Autodesk Inventor part; units mm, degrees
ref_plane "YZ Plane" through (0, 0, 0) normal (1, 0, 0) x (0, 1, 0)
ref_plane "XZ Plane" through (0, 0, 0) normal (0, 1, 0) x (-1, 0, 0)
ref_plane "XY Plane" through (0, 0, 0) normal (0, 0, 1) x (1, 0, 0)
sketch "Sketch1" plane through (0, 0, 0) normal (0, 1, 0) x (-1, 0, 0)
  line L0 (7.98, 15.9) -> (-7.98, 15.9)
  line L1 (-7.98, 15.9) -> (-7.98, -15.9)
  line L2 (-7.98, -15.9) -> (7.98, -15.9)
  line L3 (7.98, -15.9) -> (7.98, 15.9)
  line L4 (7.98, 15.9) -> (-7.98, -15.9) construction
  line L5 (-7.98, 15.9) -> (7.98, -15.9) construction
  point P0 (0, 0)
  dimension "d0" = 31.8
  dimension "d1" = 15.96
extrude "adapter-arm" add sketch "Sketch1" along normal blind 6
sketch "fanslot" plane through (0, 6, 0) normal (0, 1, 0) x (1, 0, 0)
  line L0 (-4.8, -15.9) -> (4.8, -15.9)
  line L1 (4.8, -15.9) -> (5.5, 15.9)
  line L2 (5.5, 15.9) -> (-5.5, 15.9)
  line L3 (-5.5, 15.9) -> (-4.8, -15.9)
  line L4 (0, 16.157) -> (0, -15.9695) construction
  line L5 (-7.98, -15.9) -> (7.98, -15.9) construction
  line L6 (7.98, 15.9) -> (-7.98, 15.9) construction
  point P0 (0, 0)
  point P1 (0, -15.9)
  point P2 (0, 15.9)
  point P3 (-5.98, -15.9)
  point P4 (5.98, -15.9)
  point P5 (5.98, 15.9)
  point P6 (-5.98, 15.9)
  dimension "d21" = 11
  dimension "d22" = 9.6
extrude "Extrusion3" cut sketch "fanslot" against normal blind 2
sketch "Sketch5" plane through (0, 0, 0) normal (0, -1, 0) x (1, 0, 0)
  circle A0 centre (0, 0) radius 2.5
  dimension "d25" = 5
extrude "Extrusion4" cut sketch "Sketch5" against normal up to next
sketch "Sketch6" plane through (-7.98, 0, 15.9) normal (0, 0, 1) x (1, 0, 0)
  line L0 (15.96, 0) -> (17.76, 0)
  line L1 (17.76, 0) -> (17.76, 0.8)
  line L2 (17.76, 0.8) -> (15.96, 0.8)
  line L3 (15.96, 0.8) -> (15.96, 0)
  line L4 (0, 0) -> (-1.8, 0)
  line L5 (-1.8, 0) -> (-1.8, 0.8)
  line L6 (-1.8, 0.8) -> (0, 0.8)
  line L7 (0, 0.8) -> (0, 0)
  point P0 (7.98, 0)
  dimension "d28" = 1.8
  dimension "d29" = 0.8
  dimension "d30" = 1.8
  dimension "d31" = 0.8
extrude "Extrusion5" add sketch "Sketch6" against normal up to surface (31.8 mm away)
equation "\"d2\" = adapterwallthick"
equation "\"d21\" = fanhb"
equation "\"d22\" = fanhs"
equation "\"d23\" = adapterwallslotd"
equation "\"printer3dtolerance\" = 0.1"
equation "\"wallw\" = 42"
equation "\"wallh\" = 44"
equation "\"cornerrad\" = 2"
equation "\"baseextra\" = 2"
equation "\"wall1_thick\" = 8"
equation "\"wall2_thick\" = 6.4"
equation "\"wall3_thick\" = 4"
equation "\"wall1slot\" = 8.1"
equation "\"wall2slot\" = 6.5"
equation "\"wall3slot\" = 4.1"
equation "\"gap2\" = 28"
equation "\"baseh\" = 79"
equation "\"basew\" = 44"
equation "\"base_thick\" = 6"
equation "\"base_slots_depth\" = 4"
equation "\"servobigcircledia\" = 11.6"
equation "\"servosmallcircledia\" = 5.9"
equation "\"servo9gw\" = 22.8"
equation "\"servomounth\" = 4"
equation "\"servomountsquare\" = 4"
equation "\"servopolygonr\" = 6.1"
equation "\"servopolygonl\" = 5.9"
equation "\"distancefrombottom\" = 34"
equation "\"distancefromleft\" = 22"
equation "\"wall3slotd\" = 2"
equation "\"wall3slotw\" = 36"
equation "\"adapterh\" = 16"
equation "\"adapterw\" = 32"
equation "\"armw\" = 34"
equation "\"armslotd\" = 2"
equation "\"armthick\" = 3"
equation "\"fanhb\" = 11"
equation "\"fanhs\" = 9.6"
equation "\"adapterwallthick\" = 6"
equation "\"adapterwallslotd\" = 2"
equation "\"hornscrewheadd\" = 3"
equation "\"hornscrewholed\" = 2"
equation "\"hornthick\" = 1.5"
equation "\"armhornthick\" = 3"
properties part number "adapter-wall"
Check sheet for the modelled part. Datum: model origin and axes. Units: mm. A direction names the side the tool comes from. Round coordinates to 2 decimals unless told otherwise and drop trailing zeros. Order: outer loops, then holes, each group sorted by start corner. A loop starts at its lowest first (then second) coordinate and runs counter-clockwise, first axis right, second up.
Q1. Set-up check for faces 1 (the face through (7.98, 3, 0)), 2 (the face through (-9, 0.8, 0)): record each of +Z, -Z, +X, -X, +Y, -Y from which the full face is reachable in a straight line by a thin tool's end or side.
Filled sheet:
face 1: +Z, -Z, +X, +Y
face 2: +Z, -Z, -X, +Y
Q2. Cross-section at C-C, the plane x = 0.25. Enter the section's corners in (y, z), plus the area to 3 significant figures.
Filled sheet:
outline: (0, -15.9) - (4, -15.9) - (4, -2.49) - (0, -2.49) - close; (0, 2.49) - (4, 2.49) - (4, 15.9) - (0, 15.9) - close
area: 107 mm2
Q3. Cross-section at D-D, the plane y = 2.8. Enter the section's corners in (x, z), plus the area to 3 significant figures.
Filled sheet:
outline: (-7.98, -15.9) - (7.98, -15.9) - (7.98, 15.9) - (-7.98, 15.9) - close; hole circle Ø5 at (0, 0)
area: 488 mm2
Q4. Depth check by flat-ended pin: P1, Ø3, axis at y = 4.5, z = 11.5, coming from the +X side; P2, Ø0.9, axis at x = 9, z = -3.5, coming from the +Y side; P3, Ø1, axis at x = -1.5, z = -3, coming from the -Y side; P4, Ø6, axis at x = 0, z = 0, coming from the +Y side. Enter the tip coordinate at first touch or a pass-through.
Filled sheet:
P1: stops at x = 7.98
P2: stops at y = 0.8
P3: stops at y = 0
P4: stops at y = 4
Q5. Scan lines: L1, parallel to Z at x = 0, y = 2.1; L2, parallel to X at y = 2.65, z = -10; L3, parallel to Y at x = 8.75, z = 11. Record each from-to range of solid material in increasing order.
Filled sheet:
L1: z = -15.9 to -2.5, 2.5 to 15.9
L2: x = -7.98 to 7.98
L3: y = 0 to 0.8
Q6. Cross-section at A-A, the plane y = 4.35. Enter the section's corners in (x, z), plus the area to 3 significant figures.
Filled sheet:
outline: (-7.98, -15.9) - (-5.5, -15.9) - (-4.8, 15.9) - (-7.98, 15.9) - close; (4.8, 15.9) - (5.5, -15.9) - (7.98, -15.9) - (7.98, 15.9) - close
area: 180 mm2
Q7. Draft check along Z on faces 3 (the face through (-0.54, 1.97, -2.44)), 4 (the face through (0, 2, -15.9)), 5 (the face through (-6, 6, 0)). Enter one of: pulls with the +Z half, pulls with the -Z half, needs draft (parallel to the pull), parting line crosses it, or undercut.
Filled sheet:
face 3: undercut
face 4: pulls with the -Z half
face 5: needs draft
Q8. Cross-section at B-B, the plane z = 0. Enter the section's corners in (x, y), plus the area to 3 significant figures.
Filled sheet:
outline: (-9.78, 0) - (-2.5, 0) - (-2.5, 4) - (-5.15, 4) - (-5.15, 6) - (-7.98, 6) - (-7.98, 0.8) - (-9.78, 0.8) - close; (2.5, 0) - (9.78, 0) - (9.78, 0.8) - (7.98, 0.8) - (7.98, 6) - (5.15, 6) - (5.15, 4) - (2.5, 4) - close
area: 58.0 mm2
